Geometry: final body of the model. Coordinates: model frame, mm. Give positions to 0.01 mm unless a question says otherwise; leave off trailing zeros. Write each loop counter-clockwise with the first axis right and the second up, starting at its lowest first coordinate (ties: lowest second). Pieces come first, ordered by that corner, then holes. Notation, with made-up numbers: (-33, -16) -> (7, -16) arc R12 cw to (7, 6) -> close; hole circle Ø11 at (-7, -5.75). An arc over 180 degrees is marked (long way). Answer as a JSON object with one key per item and string values.
from build123d import *

# Parameters (mm, degrees)
BOSS_EXTRUDE1_DEPTH = 8.5


with BuildPart() as part:
    # Sketch1 → Boss-Extrude1 (new body)
    with BuildSketch(Plane(origin=(0, 0, 0), x_dir=(1, 0, 0), z_dir=(0, 1, 0))):
        Polygon((-0.2, 7.2), (5, 7.2), (5, 12), (-5, 12), (-5, -20), (52.5, -20), (52.5, -0.2), (-0.2, -0.2), align=None)
        Polygon((100, 12), (100, 7.2), (105.2, 7.2), (105.2, -0.2), (52.5, -0.2), (52.5, -20), (110, -20), (110, 12), align=None)
    extrude(amount=BOSS_EXTRUDE1_DEPTH)


solid = part.part
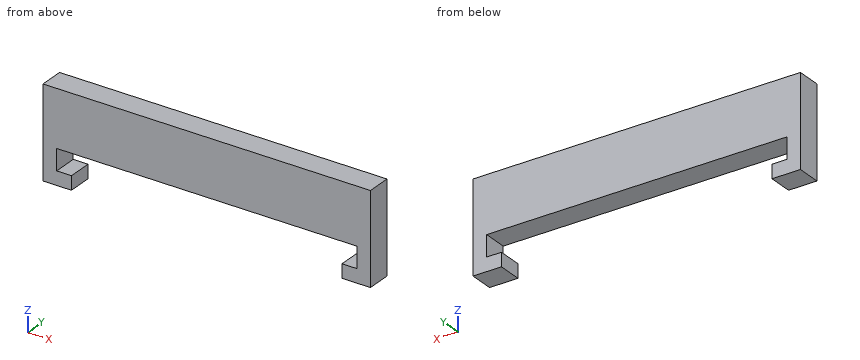
Q1. First-contact query: P1, Ø2, axis at x = 62, y = 4, coming from the -Z side. Flat tip, straight axial feed; report the tip coordinate or a pass-through.
Values:
{"P1": "z = 0.2"}
Q2. Cut plane D-D (x = 99). Return the cut outline in (y, z), and give its area (3 significant figures).
Values:
{"outline": "(0, 0.2) -> (8.5, 0.2) -> (8.5, 20) -> (0, 20) -> close", "area": "168 mm²"}
Q3. Cut plane B-B (z = -8.5). Return the cut outline in (x, y), and give its area (3 significant figures).
Values:
{"outline": "(-5, 0) -> (5, 0) -> (5, 8.5) -> (-5, 8.5) -> close; (100, 0) -> (110, 0) -> (110, 8.5) -> (100, 8.5) -> close", "area": "170 mm²"}
Q4. Cut plane C-C (y = 1). Return the cut outline in (x, z), and give its area (3 significant figures).
Values:
{"outline": "(-5, -12) -> (5, -12) -> (5, -7.2) -> (-0.2, -7.2) -> (-0.2, 0.2) -> (105.2, 0.2) -> (105.2, -7.2) -> (100, -7.2) -> (100, -12) -> (110, -12) -> (110, 20) -> (-5, 20) -> close", "area": "2,440 mm²"}
Q5. Material intervals for L1, parallel to X at y = 1, z = -7; L2, parallel to X at y = 1.5, z = -9.5; L3, parallel to Z at x = 81.5, y = 3.75, sorted ascending. Write a range as from..to.
Values:
{"L1": "-5..-0.2, 105.2..110", "L2": "-5..5, 100..110", "L3": "0.2..20"}
Q6. Cut plane A-A (x = 3). Return the cut outline in (y, z).
Values:
{"outline": "(0, -12) -> (8.5, -12) -> (8.5, -7.2) -> (0, -7.2) -> close; (0, 0.2) -> (8.5, 0.2) -> (8.5, 20) -> (0, 20) -> close"}
